```python
from build123d import *

# Parameters (mm, degrees)
CUT_EXTRUDE_1_REACH = 72.014
SKETCH_2_R          = 1.5
CHAMFER_1_SIZE      = 1.5
CUT_EXTRUDE_2_REACH = 72.014
SKETCH_3_R          = 1.5
CHAMFER_2_SIZE      = 0.5


with BuildPart() as part:
    # 草图1 → 旋转1 (revolve)
    with BuildSketch(Plane.XY, mode=Mode.PRIVATE) as revolve_1_sk:
        Polygon((-62, 18), (-62, 9.5), (-60, 9.5), (-60, 16), (0, 16), (0, 23), (-3, 23), (-3, 18), align=None)
    revolve(revolve_1_sk.sketch.rotate(Axis((-69.956231489, 0, 0), (1, 0, 0)), 90), axis=Axis((-69.956231489, 0, 0), (1, 0, 0)))

    # 草图2 → 切除-拉伸1 (cut, up to next)
    with BuildSketch(Plane.ZY.offset(62), mode=Mode.PRIVATE) as cut_extrude_1_sk1:
        with Locations((0, 13)):
            Circle(SKETCH_2_R)
    cut_extrude_1_tool1 = extrude(cut_extrude_1_sk1.sketch, amount=-CUT_EXTRUDE_1_REACH, mode=Mode.PRIVATE) & part.part
    # 草图2 → 切除-拉伸1 (cut, up to next)
    with BuildSketch(Plane.ZY.offset(62), mode=Mode.PRIVATE) as cut_extrude_1_sk2:
        with Locations((13, 0)):
            Circle(SKETCH_2_R)
    cut_extrude_1_tool2 = extrude(cut_extrude_1_sk2.sketch, amount=-CUT_EXTRUDE_1_REACH, mode=Mode.PRIVATE) & part.part
    # 草图2 → 切除-拉伸1 (cut, up to next)
    with BuildSketch(Plane.ZY.offset(62), mode=Mode.PRIVATE) as cut_extrude_1_sk3:
        with Locations((0, -13)):
            Circle(SKETCH_2_R)
    cut_extrude_1_tool3 = extrude(cut_extrude_1_sk3.sketch, amount=-CUT_EXTRUDE_1_REACH, mode=Mode.PRIVATE) & part.part
    # 草图2 → 切除-拉伸1 (cut, up to next)
    with BuildSketch(Plane.ZY.offset(62), mode=Mode.PRIVATE) as cut_extrude_1_sk4:
        with Locations((-13, 0)):
            Circle(SKETCH_2_R)
    cut_extrude_1_tool4 = extrude(cut_extrude_1_sk4.sketch, amount=-CUT_EXTRUDE_1_REACH, mode=Mode.PRIVATE) & part.part
    add(cut_extrude_1_tool1.solids().sort_by_distance((-62, 13, 0))[0], mode=Mode.SUBTRACT)
    add(cut_extrude_1_tool2.solids().sort_by_distance((-62, 0, 13))[0], mode=Mode.SUBTRACT)
    add(cut_extrude_1_tool3.solids().sort_by_distance((-62, -13, 0))[0], mode=Mode.SUBTRACT)
    add(cut_extrude_1_tool4.solids().sort_by_distance((-62, 0, -13))[0], mode=Mode.SUBTRACT)

    # 倒角1
    chamfer_1_edges = [part.edges().sort_by_distance(p)[0] for p in [
        (-62, 13, -1.5),
        (-62, 0, 11.5),
        (-62, -13, -1.5),
        (-62, 0, -14.5),
    ]]
    chamfer(chamfer_1_edges, length=CHAMFER_1_SIZE)

    # 草图3 → 切除-拉伸2 (cut, up to next)
    with BuildSketch(Plane(origin=(0, 0, 0), x_dir=(0, 0, -1), z_dir=(1, 0, 0)), mode=Mode.PRIVATE) as cut_extrude_2_sk1:
        with Locations((0, 20.5)):
            Circle(SKETCH_3_R)
    cut_extrude_2_tool1 = extrude(cut_extrude_2_sk1.sketch, amount=-CUT_EXTRUDE_2_REACH, mode=Mode.PRIVATE) & part.part
    # 草图3 → 切除-拉伸2 (cut, up to next)
    with BuildSketch(Plane(origin=(0, 0, 0), x_dir=(0, 0, -1), z_dir=(1, 0, 0)), mode=Mode.PRIVATE) as cut_extrude_2_sk2:
        with Locations((20.5, 0)):
            Circle(SKETCH_3_R)
    cut_extrude_2_tool2 = extrude(cut_extrude_2_sk2.sketch, amount=-CUT_EXTRUDE_2_REACH, mode=Mode.PRIVATE) & part.part
    # 草图3 → 切除-拉伸2 (cut, up to next)
    with BuildSketch(Plane(origin=(0, 0, 0), x_dir=(0, 0, -1), z_dir=(1, 0, 0)), mode=Mode.PRIVATE) as cut_extrude_2_sk3:
        with Locations((0, -20.5)):
            Circle(SKETCH_3_R)
    cut_extrude_2_tool3 = extrude(cut_extrude_2_sk3.sketch, amount=-CUT_EXTRUDE_2_REACH, mode=Mode.PRIVATE) & part.part
    # 草图3 → 切除-拉伸2 (cut, up to next)
    with BuildSketch(Plane(origin=(0, 0, 0), x_dir=(0, 0, -1), z_dir=(1, 0, 0)), mode=Mode.PRIVATE) as cut_extrude_2_sk4:
        with Locations((-20.5, 0)):
            Circle(SKETCH_3_R)
    cut_extrude_2_tool4 = extrude(cut_extrude_2_sk4.sketch, amount=-CUT_EXTRUDE_2_REACH, mode=Mode.PRIVATE) & part.part
    add(cut_extrude_2_tool1.solids().sort_by_distance((0, 20.5, 0))[0], mode=Mode.SUBTRACT)
    add(cut_extrude_2_tool2.solids().sort_by_distance((0, 0, -20.5))[0], mode=Mode.SUBTRACT)
    add(cut_extrude_2_tool3.solids().sort_by_distance((0, -20.5, 0))[0], mode=Mode.SUBTRACT)
    add(cut_extrude_2_tool4.solids().sort_by_distance((0, 0, 20.5))[0], mode=Mode.SUBTRACT)

    # 倒角2
    chamfer_2_edges = [part.edges().sort_by_distance(p)[0] for p in [
        (0, 0, -16),
        (-62, 0, -18),
    ]]
    chamfer(chamfer_2_edges, length=CHAMFER_2_SIZE)


solid = part.part
```
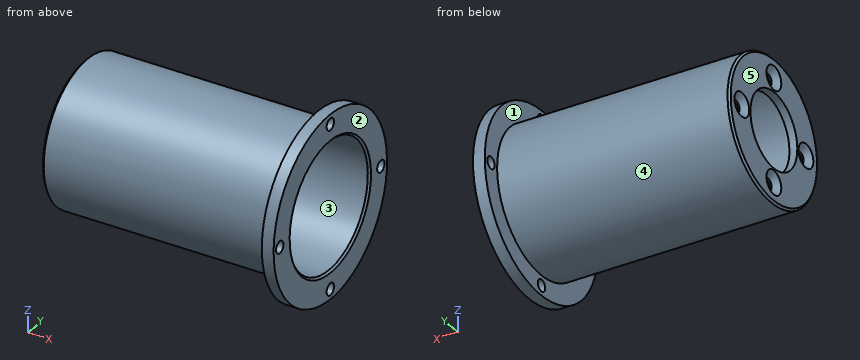
Work out the finished part from the listing and answer in its coordinate system (mm). Face numbers are marked on the shaded views. A direction names the side the tool comes from. Give positions to 0.01 mm unless a question says otherwise; leave off trailing zeros. Write each loop counter-clockwise with the first axis right and the second up, starting at its lowest first coordinate (ties: lowest second). Pieces come first, ordered by that corner, then holes. Notation, with made-up numbers: (8.5, 7) -> (66.5, 7) arc R12 ccw to (66.5, 25) -> close; hole circle Ø6 at (65.25, 52). An arc over 180 degrees is marked (long way). Write item = value, one per line.
Q1. Section B-B on x = -36 is taken. Determine the outline of the cut face in (y, z), and give its area (3 significant figures).
Computed values:
outline = circle Ø36 at (0, 0); hole circle Ø32 at (0, 0)
area = 214 mm^2
Q2. Section C-C on y = 0 is taken. State how many separate pieces and enclosed holes the cut face has, and give its area (3 significant figures).
Computed values:
separate_pieces = 6
enclosed_holes = 0
area = 269 mm^2
Q3. Section A-A on y = 20.5 is taken. Determine the outline of the cut face in (x, z).
Computed values:
outline = (-3, -10.43) -> (0, -10.43) -> (0, -1.5) -> (-3, -1.5) -> close; (-3, 1.5) -> (0, 1.5) -> (0, 10.43) -> (-3, 10.43) -> close
Q4. A tool of negligible diameter and unlimited length cuts with its end or side. For the marked faces 1 and 2, from which of +Z, -Z, +X, -X, +Y, -Y can it reach the whole face along a straight path? Write none if from no direction.
Computed values:
face_1 = -X
face_2 = +Z, -Z, +X, +Y, -Y
Q5. Consider line 1 along X through (y, z) = (4, 20); line 2 along Y through (x, z) = (-18, -0.5); line 3 along Y through (x, z) = (-28, -8). Determine where each line is inside the solid, lowest interval first.
Computed values:
line_1 = -3 to 0
line_2 = -17.99 to -15.99, 15.99 to 17.99
line_3 = -16.12 to -13.86, 13.86 to 16.12
Q6. Flat-ended cylindrical pins translate along their axes: pin 1 Ø1.5 at (x, z) = (-54, -2.5) entering from -Y; pin 2 Ø5 at (y, z) = (0, -13) entering from -X; pin 3 Ø1.8 at (y, z) = (-13, 0) entering from -X; pin 4 Ø6 at (x, z) = (-45, -3) entering from -Y. Find the tip coordinate at first contact, or state that the pin passes through.
Computed values:
pin_1 = -17.91
pin_2 = -61.5
pin_3 = through
pin_4 = -18
Q7. For a pull along Z with two mould halves and no side action, classify the marked faces 3, 4 and 5 as pulls with the +Z half, pulls with the -Z half, needs draft (parallel to the pull), parting line crosses it, or undercut.
Computed values:
face_3 = undercut
face_4 = parting line crosses it
face_5 = needs draft
